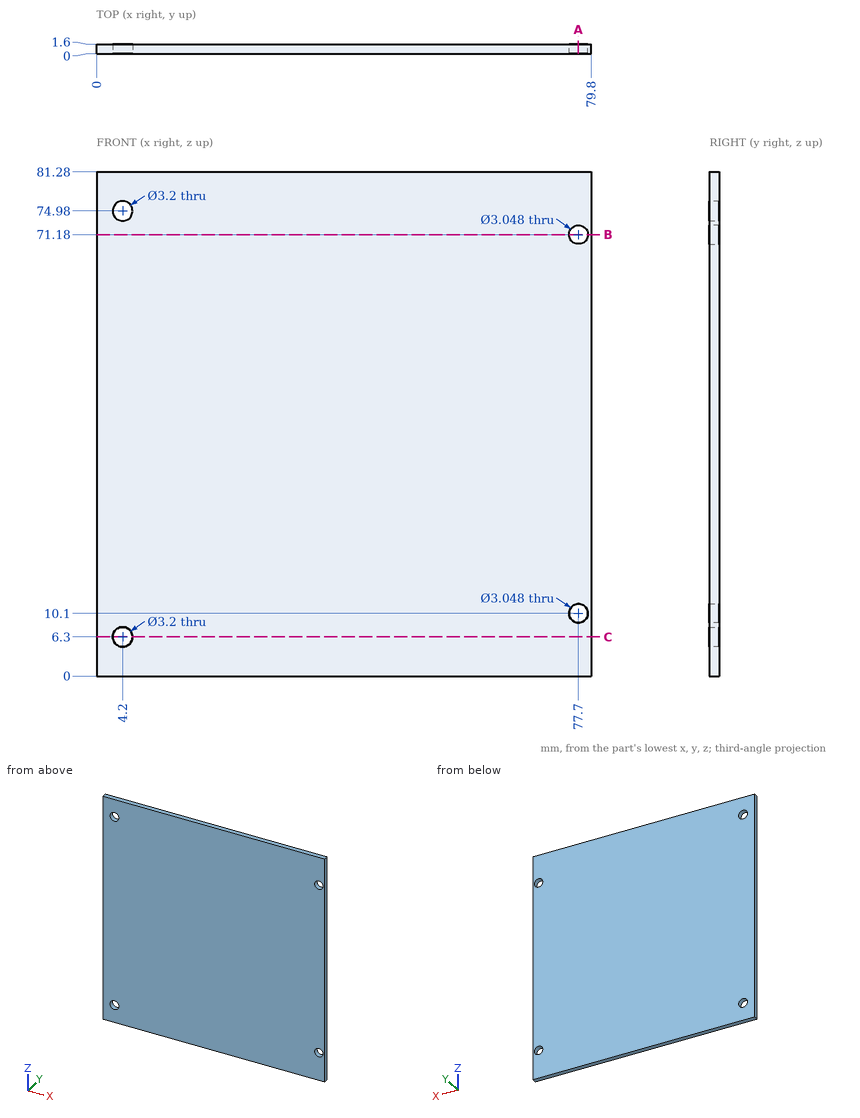
Geometry check sheet. Reference: drawing and pictorial views, mm from the part's lowest x, y, z. Round coordinates to 2 decimals unless told otherwise and drop trailing zeros. Loops run counter-clockwise (first coordinate to the right, second up) from the corner with the lowest first, then second, coordinate; pieces in that order, holes last. Notation, with made-up numbers: M -31.5,5.25 L 10.5,5.25 A17 ccw 10.5,26.25 Z; hole C 74,20 d5. An arc over 180 degrees is marked long. One line per item, written item: value.
(1) Sectioned sample at A-A, the plane x = 77.7. Record the cut outline in (y, z).
Computed values:
outline: M 0,0 L 1.6,0 L 1.6,8.58 L 0,8.58 Z; M 0,11.62 L 1.6,11.62 L 1.6,69.66 L 0,69.66 Z; M 0,72.7 L 1.6,72.7 L 1.6,81.28 L 0,81.28 Z
(2) Thickness scan on line 1 (Z direction, x = 77.7, y = 0.9); line 2 (X direction, y = 0.8, z = 6.3); line 3 (X direction, y = 1.1, z = 71.18). Record the ranges inside material, lowest first.
Computed values:
line 1: z = 0 to 8.58, 11.62 to 69.66, 72.7 to 81.28
line 2: x = 0 to 2.6, 5.8 to 79.8
line 3: x = 0 to 76.18, 79.22 to 79.8
(3) Sectioned sample at C-C, the plane z = 6.3. Record the cut outline in (x, y).
Computed values:
outline: M 0,0 L 2.6,0 L 2.6,1.6 L 0,1.6 Z; M 5.8,0 L 79.8,0 L 79.8,1.6 L 5.8,1.6 Z
(4) Sectioned sample at B-B, the plane z = 71.18. Record the cut outline in (x, y).
Computed values:
outline: M 0,0 L 76.18,0 L 76.18,1.6 L 0,1.6 Z; M 79.22,0 L 79.8,0 L 79.8,1.6 L 79.22,1.6 Z
(5) Depth check by flat-ended pin: pin 1 Ø4 at (x, z) = (4.2, 6.3) entering from +Y; pin 2 Ø3 at (x, z) = (4.2, 74.98) entering from +Y. Enter the tip coordinate at first touch or a pass-through.
Computed values:
pin 1: stops at y = 1.6
pin 2: passes through
